Geometry: see drawing. Coordinates: mm, zero at the bounding-box minimum. A direction names the side the tool comes from. Coordinates: 2 decimals unless noted, no trailing zeros. Loops run counter-clockwise (first coordinate to the right, second up) from the corner with the lowest first, then second, coordinate; pieces in that order, holes last.
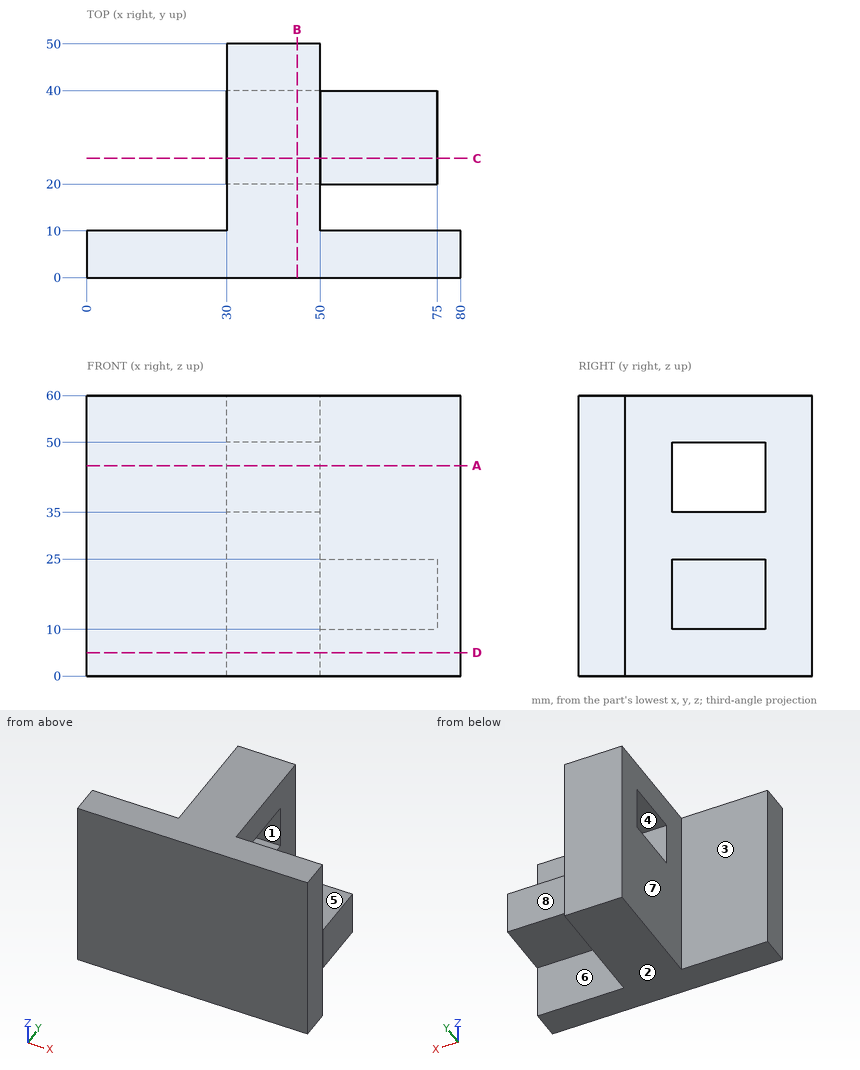
Item 1: Section query A-A (z = 45). Output: boundary loops of the cut face in (x, y), then the cut area to 3 significant figures.
Result:
outline: (0, 0) - (80, 0) - (80, 10) - (50, 10) - (50, 20) - (30, 20) - (30, 10) - (0, 10) - close; (30, 40) - (50, 40) - (50, 50) - (30, 50) - close
area: 1,200 mm2
Item 2: Line query: L1, parallel to Y at x = 54, z = 11; L2, parallel to Y at x = 48, z = 42.5; L3, parallel to Z at x = 31, y = 24.5. Output: solid intervals per line, ascending.
Result:
L1: y = 0 to 10, 20 to 40
L2: y = 0 to 20, 40 to 50
L3: z = 0 to 35, 50 to 60
Item 3: Section query D-D (z = 5). Output: boundary loops of the cut face in (x, y).
Result:
outline: (0, 0) - (80, 0) - (80, 10) - (50, 10) - (50, 50) - (30, 50) - (30, 10) - (0, 10) - close
Item 4: Reachability of the marked faces 4, 5, 6, 7 and 8 from +Z, -Z, +X, -X, +Y, -Y: full face, straight path, thin tool, end or side. Return the list, or none.
Result:
face 4: +X, -X
face 5: +Z, +X, +Y
face 6: +Z, -Z, +X
face 7: +Z, -Z, -X, +Y
face 8: +Z, -Z, +X, +Y
Item 5: Mould query, pull axis Z, two halves, no side actions, for the marked faces 1, 2 and 3. Classes: +Z half, -Z half, draft (parallel to the pull), parting line (faces both ways), or undercut.
Result:
face 1: undercut
face 2: -Z half
face 3: draft
Item 6: Section query C-C (y = 25.5). Output: boundary loops of the cut face in (x, z), then the cut area to 4 significant figures.
Result:
outline: (30, 0) - (50, 0) - (50, 10) - (75, 10) - (75, 25) - (50, 25) - (50, 35) - (30, 35) - close; (30, 50) - (50, 50) - (50, 60) - (30, 60) - close
area: 1,275 mm2
Item 7: Section query B-B (x = 45). Output: boundary loops of the cut face in (y, z), then the cut area to 3 significant figures.
Result:
outline: (0, 0) - (50, 0) - (50, 60) - (0, 60) - close; hole (20, 35) - (40, 35) - (40, 50) - (20, 50) - close
area: 2,700 mm2
Item 8: Contact query for flat-ended pins moving along their axis: P1, Ø16.5, axis at y = 26.5, z = 20, coming from the +X side; P2, Ø5, axis at x = 42, z = 19.5, coming from the -Y side; P3, Ø16, axis at x = 59, y = 29, coming from the -Z side; P4, Ø10, axis at x = 24, z = 8.5, coming from the +Y side. Output: stop coordinate, or through.
Result:
P1: stops at x = 75
P2: stops at y = 0
P3: stops at z = 10
P4: stops at y = 10
